Could you check a few things on this model? Use its own coordinates, in mm. Face numbers are marked on the shaded views. A direction names the side the tool comes from. Round coordinates to 2 decimals unless told otherwise and drop trailing zeros. Loops run counter-clockwise (first coordinate to the right, second up) from the corner with the lowest first, then second, coordinate; pieces in that order, holes last. Notation, with made-up numbers: M -33.5,65.5 L -26.5,65.5 A22 cw -26.5,71.5 Z; hole C 2.25,53 d8. An arc over 180 degrees is marked long. Return JSON: item names as keys, results as strings. Group by question number.
```python
from build123d import *

# Parameters (mm, degrees)
BOSS_EXTRUDE1_DEPTH = 15
SKETCH3_R           = 1.75
CUT_EXTRUDE1_DEPTH  = 1
CHAMFER1_SIZE       = 0.5


with BuildPart() as part:
    # Sketch2 → Boss-Extrude1 (new body)
    with BuildSketch(Plane.XY):
        with BuildLine():
            Line((0, 0), (0, 5))
            Line((0, 5), (2.7, 5))
            ThreePointArc((2.7, 5), (4, 3.7), (5.3, 5))
            Line((5.3, 5), (8, 5))
            Line((8, 5), (8, 2))
            Line((8, 2), (30, 2))
            Line((30, 2), (30, 0))
            Line((30, 0), (0, 0))
        make_face()
    extrude(amount=BOSS_EXTRUDE1_DEPTH)

    # Sketch3 → Cut-Extrude1 (cut)
    with BuildSketch(Plane.XZ):
        with Locations(Location((15, 7.5, 0), (0, 0, 270))):
            Circle(SKETCH3_R)
    extrude(amount=-CUT_EXTRUDE1_DEPTH, mode=Mode.SUBTRACT)

    # Chamfer1
    chamfer1_edges = [part.edges().sort_by_distance(p)[0] for p in [
        (15, 1, 9.25),
        (15, 0, 9.25),
    ]]
    chamfer(chamfer1_edges, length=CHAMFER1_SIZE - 0.0001)  # a hair under: the kernel refuses the full size


solid = part.part
```
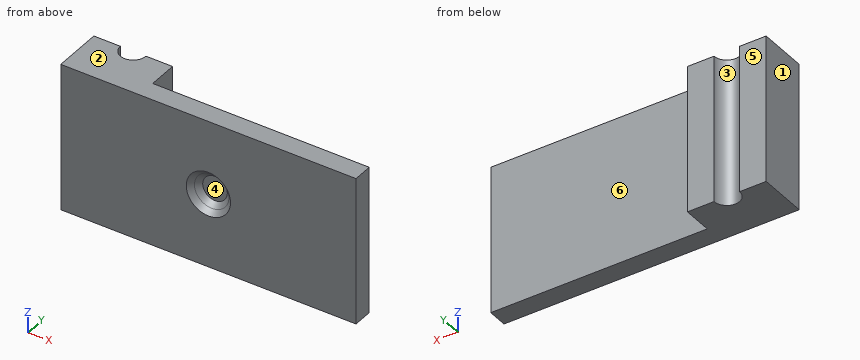
1. On a 3-axis mill with a long thin cutter (end or side, diameter ignored), from which of +Z, -Z, +X, -X, +Y, -Y can I reach the whole of each face in a straight line? I mean the marked faces 4, 5 and 6. Say none if no direction works.
2. If we section it at B-B, the plane y = 4.6: Please give me the cut outline in (x, z), then the cut area to 3 significant figures.
3. I'm going to push flat-ended pins straight in: pin 1 Ø7.5 at (x, z) = (20, 6) entering from +Y; pin 2 Ø3 at (y, z) = (4.5, 13) entering from +X; pin 3 Ø2 at (x, z) = (15, 7.5) entering from -Y. Where does each tip first touch, or does it pass through?
4. If we section it at D-D, the plane x = 23.75: Please give me the cut outline in (y, z).
5. We'd pull the mould along X, two halves only. Please class the marked faces 1, 2 and 3: +X half, -X half, draft (parallel to the pull), parting line (faces both ways), or undercut.
6. I need wall thicknesses on probe 1 along X at (y, z) = (0.5, 7.5); probe 2 along Y at (x, z) = (26.5, 5.25); probe 3 along Z at (x, y) = (15, 0.55). Which ranges of each line are inside material? Lowest first, please.
Geometry results:
{
 "1": {"face 4": "-Y", "face 5": "+Z, -Z, +X, -X, +Y", "face 6": "+Z, -Z, +X, +Y"},
 "2": {"outline": "M 0,0 L 2.76,0 L 2.76,15 L 0,15 Z; M 5.24,0 L 8,0 L 8,15 L 5.24,15 Z", "area": "82.9 mm^2"},
 "3": {"pin 1": "y = 2", "pin 2": "x = 8", "pin 3": "y = 1"},
 "4": {"outline": "M 0,0 L 2,0 L 2,15 L 0,15 Z"},
 "5": {"face 1": "-X half", "face 2": "draft", "face 3": "undercut"},
 "6": {"probe 1": "0 to 13.25, 16.75 to 30", "probe 2": "0 to 2", "probe 3": "0 to 5.8, 9.2 to 15"}
}
